Solid Edge part; units mm, degrees
sketch "Sketch1" plane through (0, 0, 0) normal (0, 0, 1) x (1, 0, 0)
  line L0 (-0.0293, -36.1666) -> (31.3359, 18.0579)
  line L1 (31.3359, 18.0579) -> (-31.3066, 18.1087)
  line L2 (-31.3066, 18.1087) -> (-0.0293, -36.1666)
extrude "Protrusion1" add sketch "Sketch1" along normal blind 50.788
sketch "Sketch2" plane through (0, 0, 0) normal (1, 0, 0) x (0, 1, 0)
  line L0 (0, 51.1801) -> (18.0579, 0)
extrude "ExtrudedCutout_14" cut sketch "Sketch2" along normal mid plane 199.174 material side at (0, 9.0761, 25.6067)
pattern_circular "Pattern1" count 3 over 360 about axis through (0, 0, 0) along (0, 0, 1) of "ExtrudedCutout_14"
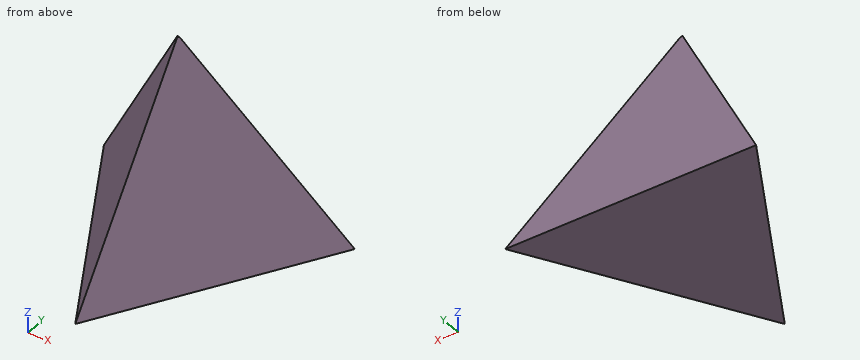
Source: CAD feature listing. Evaluate the final solid. Frame: model axes, mm. Round coordinates to 2 decimals unless told otherwise and drop trailing zeros. Loops run counter-clockwise (first coordinate to the right, second up) from the corner with the lowest first, then second, coordinate; pieces in that order, holes last. Notation, with made-up numbers: M 3.5,40.25 L 12.5,40.25 A23 ccw 12.5,79.25 Z; hole C -7,-15.5 d5. An arc over 180 degrees is marked long. Put each result on its own line as item: value.
(1) Section B-B, the plane y = 5. Return loops of the section in (x, z), and give its area (3 significant figures).
Solutions:
outline: M -23.74,0 L 23.74,0 L 8.66,37.01 L -8.66,37.01 Z
area: 1,200 mm²
(2) Section A-A, the plane z = 30. Return loops of the section in (x, y), and give its area (3 significant figures).
Solutions:
outline: M -12.94,7.47 L 0,-14.95 L 12.94,7.47 Z
area: 290 mm²
(3) First-contact query: pin 1 (6 mm diameter, centred on y = -8.5, z = 10.5, fed in from +X); pin 2 (1 mm diameter, centred on y = -23.5, z = 5.5, fed in from -X); pin 3 (12 mm diameter, centred on y = 9, z = 12, fed in from +X); pin 4 (12 mm diameter, centred on x = 17.5, z = 37.5, fed in from +Y). Flat tips, straight axial feed; report the tip coordinate or a pass-through.
Solutions:
pin 1: x = 13.79
pin 2: x = -5.4
pin 3: x = 25.4
pin 4: through
(4) Ray query, line 1 (Y direction, x = -12, z = 26.5); line 2 (Z direction, x = 2.5, y = -3); line 3 (X direction, y = -26, z = 2). Return the intervals inside material, ascending. Write a range as [from, to].
Solutions:
line 1: [3.37, 8.71]
line 2: [0, 40.79]
line 3: [-5.03, 5.03]
(5) Section C-C, the plane x = -20.5. Return loops of the section in (y, z).
Solutions:
outline: M -0.61,0 L 18.06,0 L 11.84,17.64 Z
